CAD build for the part. Positions are in the model's coordinates, mm. Coordinates: 2 decimals unless noted, no trailing zeros. Write each loop counter-clockwise with the first axis right and the second up, starting at its lowest first coordinate (ties: lowest second). Pieces come first, ordered by that corner, then holes. Notation, with made-up numbers: M 22,-40 L 35,-40 A22 ccw 35,-1 Z; hole C 68,25 d5. An arc over 180 degrees is marked long. Put each result on its own line as item: value. Start each with the question number.
```python
from build123d import *

# Parameters (mm, degrees)
BOSS_EXTRUDE1_DEPTH      = 0.79375
BOSS_EXTRUDE1_DEPTH_BACK = 0.79375
SKETCH1_W                = 75
SKETCH1_H                = 62.5
SKETCH1_R                = 13.5
SKETCH1_R_2              = 2.6


with BuildPart() as part:
    # Sketch1 → Boss-Extrude1 (new, two sides: drawn at the far end of the back side and taken through both)
    with BuildSketch(Plane(origin=(0, 0, 0), x_dir=(1, 0, 0), z_dir=(0, 1, 0)).offset(-BOSS_EXTRUDE1_DEPTH_BACK)):
        Rectangle(SKETCH1_W, SKETCH1_H)
        with Locations(Location((0, 0, 0), (0, 0, 270))):
            Circle(SKETCH1_R, mode=Mode.SUBTRACT)
        with Locations(Location((30, 25, 0), (0, 0, 270))):
            Circle(SKETCH1_R_2, mode=Mode.SUBTRACT)
        with Locations(Location((-30, 25, 0), (0, 0, 90))):
            Circle(SKETCH1_R_2, mode=Mode.SUBTRACT)
        with Locations(Location((30, -25, 0), (0, 0, 90))):
            Circle(SKETCH1_R_2, mode=Mode.SUBTRACT)
        with Locations(Location((-30, -25, 0), (0, 0, 270))):
            Circle(SKETCH1_R_2, mode=Mode.SUBTRACT)
    extrude(amount=BOSS_EXTRUDE1_DEPTH + BOSS_EXTRUDE1_DEPTH_BACK)


solid = part.part
```
(1) Slice it at B-B, the plane z = 0. Write the cut outline in (x, y).
(2) Two-plate mould, pull along X, no slides. Class faces 1 (the face through (37.5, 0, 0)), 2 (the face through (-29.22, -0.01, 27.48)), 3 (the face through (29.22, -0.01, 22.52)), 4 (the face through (-37.5, 0, 0)): +X half, -X half, draft (parallel to the pull), parting line (faces both ways), or undercut.
(3) Drop flat-ended pins along their axis: pin 1 (7 mm diameter, centred on x = 30, z = -25, fed in from -Y); pin 2 (16 mm diameter, centred on x = 0, z = 0, fed in from -Y). Give the stop position or say it passes through.
(4) Slice it at D-D, the plane y = 0.2. Write the cut outline in (x, z).
(5) Slice it at C-C, the plane x = 30. Write the cut outline in (y, z), then the cut area to 3 significant figures.
(6) Slice it at A-A, the plane z = 25. Write the cut outline in (x, y).
(7) Drill centre lines: line 1 (X direction, y = -0.35, z = -25); line 2 (X direction, y = -0.2, z = 0); line 3 (Z direction, x = 11.5, y = -0.2). Where is each one in solid material? Low to high. Write a range as [from, to].
Result set:
1. outline: M -37.5,-0.79 L -13.5,-0.79 L -13.5,0.79 L -37.5,0.79 Z; M 13.5,-0.79 L 37.5,-0.79 L 37.5,0.79 L 13.5,0.79 Z
2. face 1: +X half
2. face 2: undercut
2. face 3: undercut
2. face 4: -X half
3. pin 1: stops at y = -0.79
3. pin 2: passes through
4. outline: M -37.5,-31.25 L 37.5,-31.25 L 37.5,31.25 L -37.5,31.25 Z; hole C -30,-25 d5.2; hole C -30,25 d5.2; hole C 0,0 d27; hole C 30,-25 d5.2; hole C 30,25 d5.2
5. outline: M -0.79,-31.25 L 0.79,-31.25 L 0.79,-27.6 L -0.79,-27.6 Z; M -0.79,-22.4 L 0.79,-22.4 L 0.79,22.4 L -0.79,22.4 Z; M -0.79,27.6 L 0.79,27.6 L 0.79,31.25 L -0.79,31.25 Z
5. area: 82.7 mm^2
6. outline: M -37.5,-0.79 L -32.6,-0.79 L -32.6,0.79 L -37.5,0.79 Z; M -27.4,-0.79 L 27.4,-0.79 L 27.4,0.79 L -27.4,0.79 Z; M 32.6,-0.79 L 37.5,-0.79 L 37.5,0.79 L 32.6,0.79 Z
7. line 1: x = [-37.5, -32.6], [-27.4, 27.4], [32.6, 37.5]
7. line 2: x = [-37.5, -13.5], [13.5, 37.5]
7. line 3: z = [-31.25, -7.07], [7.07, 31.25]
